Part model, mm, in its own coordinate system. Give positions to 0.01 mm unless a question says otherwise; leave off trailing zeros. Order: outer loops, then holes, each group sorted by start corner. A loop starts at its lowest first (then second) coordinate and runs counter-clockwise, first axis right, second up. Notation, with made-up numbers: M 54,27 L 68,27 A18 ccw 68,36 Z; hole C 32.25,41 d1. An arc over 180 degrees is marked long. One line per question, with ' | ' between items.
Autodesk Inventor part; units mm, degrees
ref_plane "YZ Plane" through (0, 0, 0) normal (1, 0, 0) x (0, 1, 0)
ref_plane "XZ Plane" through (0, 0, 0) normal (0, 1, 0) x (-1, 0, 0)
ref_plane "XY Plane" through (0, 0, 0) normal (0, 0, 1) x (1, 0, 0)
sketch "Sketch1" plane through (0, 0, 0) normal (0, 1, 0) x (-1, 0, 0)
  line L0 (-31.6431, 25.3606) -> (38.3569, 25.3606)
  line L1 (100.8569, -14.6394) -> (100.8569, -54.6394)
  line L2 (-31.6431, -94.6394) -> (38.3569, -94.6394)
  arc A0 (-36.6431, -89.6394) -> (-31.6431, -94.6394) centre (-31.6431, -89.6394) ccw
  line L3 (-36.6431, -89.6394) -> (-36.6431, 20.3606)
  arc A1 (-31.6431, 25.3606) -> (-36.6431, 20.3606) centre (-31.6431, 20.3606) ccw
  circle A2 centre (-30.6431, 10.3606) radius 1.5
  circle A3 centre (45.8569, -54.6394) radius 1.25
  circle A4 centre (45.8569, -14.6394) radius 1.25
  circle A5 centre (85.8569, -14.6394) radius 1.25
  circle A6 centre (93.8569, -14.6394) radius 1.5
  circle A7 centre (93.8569, -54.6394) radius 1.5
  circle A8 centre (85.8569, -54.6394) radius 1.25
  circle A9 centre (-30.6431, -79.6394) radius 1.5
  line L4 (38.3569, -94.6394) -> (95.8569, -94.6394)
  line L5 (100.8569, -89.6394) -> (100.8569, 20.3606)
  line L6 (95.8569, 25.3606) -> (38.3569, 25.3606)
  arc A10 (95.8569, -94.6394) -> (100.8569, -89.6394) centre (95.8569, -89.6394) ccw
  arc A11 (100.8569, 20.3606) -> (95.8569, 25.3606) centre (95.8569, 20.3606) ccw
  line L7 (45.8569, -89.6394) -> (60.8569, -89.6394)
  line L8 (60.8569, -89.6394) -> (60.8569, -79.0394)
  line L9 (60.8569, -79.0394) -> (45.8569, -79.0394)
  line L10 (45.8569, -79.0394) -> (45.8569, -89.6394)
  line L11 (85.8569, -89.6394) -> (70.8569, -89.6394)
  line L12 (70.8569, -89.6394) -> (70.8569, -79.0394)
  line L13 (70.8569, -79.0394) -> (85.8569, -79.0394)
  line L14 (85.8569, -79.0394) -> (85.8569, -89.6394)
  line L15 (45.8569, 25.3606) -> (45.8569, 20.3606)
  line L16 (45.8569, 20.3606) -> (60.8569, 20.3606)
  line L17 (60.8569, 20.3606) -> (60.8569, 9.7606)
  line L18 (60.8569, 9.7606) -> (45.8569, 9.7606)
  line L19 (45.8569, 9.7606) -> (45.8569, 20.3606)
  line L20 (85.8569, 20.3606) -> (70.8569, 20.3606)
  line L21 (70.8569, 20.3606) -> (70.8569, 9.7606)
  line L22 (70.8569, 9.7606) -> (85.8569, 9.7606)
  line L23 (85.8569, 9.7606) -> (85.8569, 20.3606)
  line L24 (60.8569, -79.0394) -> (58.0285, -81.8678)
  line L25 (60.8569, -79.0394) -> (64.8569, -79.0394) construction
  line L26 (70.8569, -79.0394) -> (73.6853, -81.8678)
  line L27 (60.8569, 9.7606) -> (58.0285, 12.589)
  line L28 (60.8569, 9.7606) -> (64.8569, 9.7606) construction
  line L29 (70.8569, 9.7606) -> (73.6853, 12.589)
  line L30 (70.8569, 9.7606) -> (74.8569, 9.7606) construction
  circle A12 centre (58.0285, 12.589) radius 1.25
  circle A13 centre (73.6853, 12.589) radius 1.25
  circle A14 centre (73.6853, -81.8678) radius 1.25
  circle A15 centre (58.0285, -81.8678) radius 1.25
  point P0 (0, 0)
  point P1 (-36.6431, -94.6394)
  point P2 (-36.6431, -94.6394)
  point P3 (-36.6431, -94.6394)
  point P4 (100.8569, 25.3606)
  dimension "d8" = 5
  dimension "d9" = 15
  dimension "d10" = 10.6
  dimension "d11" = 15
  dimension "d12" = 10.6
  dimension "d13" = 5
  dimension "d14" = 5
  dimension "d15" = 15
  dimension "d16" = 10.6
  dimension "d17" = 15
  dimension "d18" = 10.6
  dimension "d19" = 4
  dimension "d20" = 135
  dimension "d21" = 4
  dimension "d22" = 4
  dimension "d23" = 135
  dimension "d24" = 4
  dimension "d25" = 45
  dimension "d26" = 2.5
  dimension "d27" = 2.5
  dimension "d28" = 2.5
  dimension "d29" = 2.5
ref_plane "Work Plane1" through (0, 3, 0) normal (0, 1, 0) x (1, 0, 0)
sketch "Sketch2" plane through (0, 3, 0) normal (0, 1, 0) x (1, 0, 0)
  circle A0 centre (16.7477, 6.3332) radius 1.25
  circle A1 centre (-32.2523, 6.3332) radius 1.25
  circle A2 centre (-32.2523, 64.3332) radius 1.25
  circle A3 centre (16.7477, 64.3332) radius 1.25
  circle A4 centre (16.7477, 64.3332) radius 1.5
  circle A5 centre (-32.2523, 64.3332) radius 1.5
  circle A6 centre (-32.2523, 6.3332) radius 1.5
  circle A7 centre (16.7477, 6.3332) radius 1.5
  point P0 (0, 0)
  dimension "d2" = 3
  dimension "d3" = 3
  dimension "d4" = 3
  dimension "d5" = 3
extrude "Extrusion3" add sketch "Sketch1" along normal blind 3 contours L16 L17 L18 L19 | L0 L6 A11 L5 L1 A10 L4 L2 A0 L3 A1 | L10 L9 L8 L7 | L11 L12 L13 L14 | L23 L22 L21 L20
extrude "Extrusion4" cut sketch "Sketch2" against normal blind 3 contours A0 | A1 | A2 | A3 | A4 | A5 | A6 | A7
sketch "Sketch3" plane through (0, 3, 0) normal (0, 1, 0) x (1, 0, 0)
  circle A0 centre (-85.8569, 14.6394) radius 1.25 construction
  circle A1 centre (-45.8569, 54.6394) radius 1.25 construction
  line L0 (-85.8569, 14.6394) -> (-45.8569, 54.6394) construction
  circle A2 centre (-85.8569, 54.6394) radius 1.25 construction
  line L1 (-85.8569, 54.6394) -> (-45.8569, 14.6394) construction
  line L2 (-80.8569, 19.6394) -> (-50.8569, 19.6394)
  line L3 (-50.8569, 19.6394) -> (-50.8569, 49.6394)
  line L4 (-50.8569, 49.6394) -> (-80.8569, 49.6394)
  line L5 (-80.8569, 49.6394) -> (-80.8569, 19.6394)
  line L6 (-80.8569, 19.6394) -> (-50.8569, 49.6394) construction
  line L7 (-50.8569, 19.6394) -> (-80.8569, 49.6394) construction
  point P0 (0, 0)
  point P1 (-65.8569, 34.6394)
  dimension "d34" = 30
  dimension "d35" = 30
extrude "Extrusion5" cut sketch "Sketch3" against normal blind 10
properties part number "Top base 2"
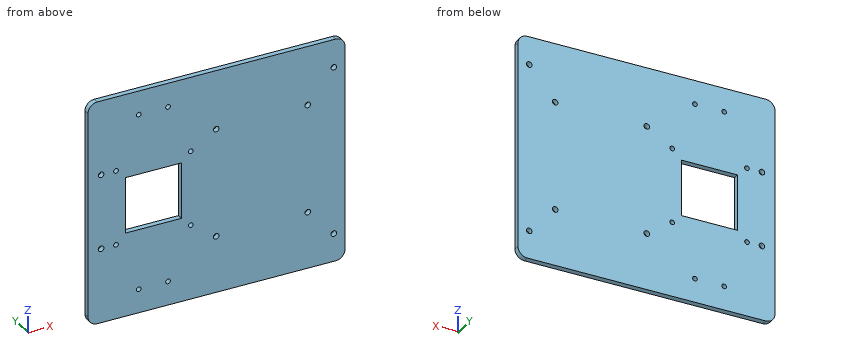
1. Drop a flat-ended pin along its axis: pin 1 (2.5 mm diameter, centred on x = -32.25, z = -6.33, fed in from +Y) (3 decimals). Give the stop position or say it passes through.
Worked out:
pin 1: passes through
2. Probe L1, parallel to Z at x = -70, y = 0.45; L2, parallel to X at y = 2.4, z = -39.5; L3, parallel to X at y = 0.65, z = -63.5 (3 decimals). List the from-to ranges inside material, lowest first. Write a range as from..to.
Worked out:
L1: z = -94.64..-49.64, -19.64..25.36 | L2: x = -100.86..-80.86, -50.86..36.64 | L3: x = -100.857..-33.5, -31.005..15.5, 17.995..36.643
3. Slice it at C-C on y = 2.05. Give the number of separate pieces and of enclosed holes in the cut face, then the cut area to 3 significant figures.
Worked out:
separate pieces: 1 | enclosed holes: 17 | area: 15,500 mm2
4. Slice it at B-B on z = -29.5. Give the cut face in (x, y), then the cut area to 4 significant figures.
Worked out:
outline: M -100.86,0 L -80.86,0 L -80.86,3 L -100.86,3 Z; M -50.86,0 L 36.64,0 L 36.64,3 L -50.86,3 Z | area: 322.5 mm2
5. Slice it at A-A on x = -78.5. Give the cut face in (y, z).
Worked out:
outline: M 0,-94.64 L 3,-94.64 L 3,-49.64 L 0,-49.64 Z; M 0,-19.64 L 3,-19.64 L 3,25.36 L 0,25.36 Z
